Geometry check sheet. Reference: the model listing, model coordinates, mm. Face numbers are marked on the shaded views. A direction names the side the tool comes from. Round coordinates to 2 decimals unless told otherwise and drop trailing zeros. Write each loop counter-clockwise with the first axis right and the second up, starting at its lowest first coordinate (ties: lowest second). Pieces come first, ordered by that corner, then holes. Notation, with made-up numbers: (-28.5, -38.5) -> (15.5, -38.5) arc R14 cw to (15.5, -24.5) -> close; hole circle Ø7 at (28.25, -5). An arc over 180 degrees is marked (long way). Return JSON: item names as keys, results as strings. Group by question number.
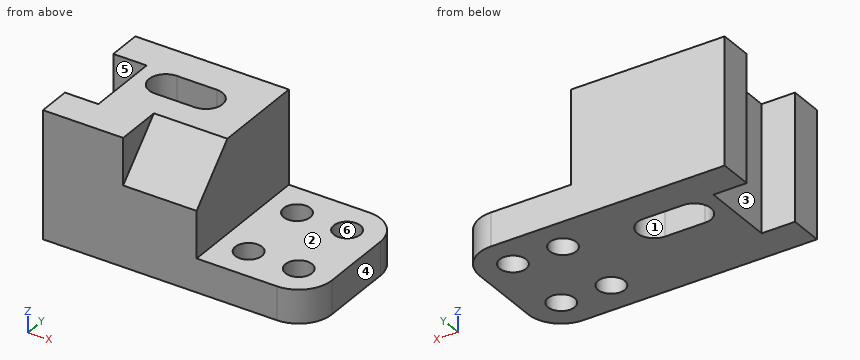
from build123d import *

# Parameters (mm, degrees)
SKETCH_W        = 80
SKETCH_H        = 42
PAD_DEPTH       = 38
SKETCH001_W     = 34
SKETCH001_H     = 42
POCKET_DEPTH    = 28
SKETCH002_W     = 10
SKETCH002_H     = 22
POCKET001_DEPTH = 38
SKETCH003_R     = 4
POCKET002_DEPTH = 38
POCKET003_DEPTH = 38
POCKET004_DEPTH = 22
FILLET_R        = 10
FILLET001_R     = 10


with BuildPart() as part:
    # Sketch → Pad (new body)
    with BuildSketch(Plane.XY):
        with Locations((40, 21)):
            Rectangle(SKETCH_W, SKETCH_H)
    extrude(amount=PAD_DEPTH)

    # Sketch001 (on Face6 of Pad) → Pocket (cut)
    with BuildSketch(Plane.XY.offset(38)):
        with Locations((63, 21)):
            Rectangle(SKETCH001_W, SKETCH001_H)
    extrude(amount=-POCKET_DEPTH, mode=Mode.SUBTRACT)

    # Sketch002 (on Face6 of Pocket) → Pocket001 (cut)
    with BuildSketch(Plane.XY.offset(38)):
        with Locations((5, 21)):
            Rectangle(SKETCH002_W, SKETCH002_H)
    extrude(amount=-POCKET001_DEPTH, mode=Mode.SUBTRACT)

    # Sketch003 (on Face6 of Pocket001) → Pocket002 (cut)
    with BuildSketch(Plane.XY.offset(38)):
        with Locations((55, 32)):
            Circle(SKETCH003_R)
        with Locations((70, 32)):
            Circle(SKETCH003_R)
        with Locations((55, 10)):
            Circle(SKETCH003_R)
        with Locations((70, 10)):
            Circle(SKETCH003_R)
    extrude(amount=-POCKET002_DEPTH, mode=Mode.SUBTRACT)

    # Sketch004 (on Face6 of Pocket002) → Pocket003 (cut)
    with BuildSketch(Plane.XY.offset(38)):
        with BuildLine():
            ThreePointArc((19, 32), (14, 27), (19, 22))
            Line((19, 22), (31, 22))
            ThreePointArc((31, 22), (35.99997, 27), (31, 32))
            Line((19, 32), (31, 32))
        make_face()
    extrude(amount=-POCKET003_DEPTH, mode=Mode.SUBTRACT)

    # Sketch005 (on Face5 of Pocket003) → Pocket004 (cut)
    with BuildSketch(Plane.YZ.offset(46)):
        Polygon((0, 24), (0, 38), (14, 38), align=None)
    extrude(amount=-POCKET004_DEPTH, mode=Mode.SUBTRACT)

    # Fillet
    fillet_edges = [part.edges().sort_by_distance(p)[0] for p in [
        (80, 0, 5),
    ]]
    fillet(fillet_edges, radius=FILLET_R)

    # Fillet001
    fillet001_edges = [part.edges().sort_by_distance(p)[0] for p in [
        (80, 42, 5),
    ]]
    fillet(fillet001_edges, radius=FILLET001_R)


solid = part.part
1) Sectioned sample at A-A on z = 11.5. Enter the section's corners in (x, y), and give its area (3 significant figures).
2) Sectioned sample at B-B on x = 55. Enter the section's corners in (y, z).
3) Sectioned sample at C-C on y = 27. Enter the section's corners in (x, z).
4) Sectioned sample at D-D on y = 20. Enter the section's corners in (x, z), and give its area (3 significant figures).
5) Tool access check on the marked faces 1, 2 and 3. Record the directions out of +Z, -Z, +X, -X, +Y, -Y that give a thin tool (end or side, any length) a straight path to the whole face; none if there is none.
6) Material ranges on probe 1 along Y at (x, z) = (70, 5); probe 2 along X at (y, z) = (11.5, 8.5); probe 3 along Z at (x, y) = (64.5, 3), recorded low to high. Write a range as [from, to].
7) Mould release check, pull along X, two halves, no side actions. Record for the marked faces 4, 5 and 6: +X half, -X half, draft (parallel to the pull), parting line (faces both ways), or undercut.
8) Go/stop test with flat-tipped pins: P1, Ø5, axis at y = 18.5, z = 20, coming from the -X side; P2, Ø12, axis at y = 21, z = 25.5, coming from the +X side; P3, Ø10.5, axis at x = 55, y = 10, coming from the +Z side. Record where each tip stops, or that it passes through.
Evaluation:
{
 "1": {"outline": "(0, 0) -> (46, 0) -> (46, 42) -> (0, 42) -> (0, 32) -> (10, 32) -> (10, 10) -> (0, 10) -> close; hole (19, 22) -> (31, 22) arc R5 ccw to (31, 32) -> (19, 32) arc R5 ccw to start", "area": "1,510 mm2"},
 "2": {"outline": "(0, 0) -> (6, 0) -> (6, 10) -> (0, 10) -> close; (14, 0) -> (28, 0) -> (28, 10) -> (14, 10) -> close; (36, 0) -> (42, 0) -> (42, 10) -> (36, 10) -> close"},
 "3": {"outline": "(10, 0) -> (14, 0) -> (14, 38) -> (10, 38) -> close; (36, 0) -> (80, 0) -> (80, 10) -> (46, 10) -> (46, 38) -> (36, 38) -> close"},
 "4": {"outline": "(10, 0) -> (80, 0) -> (80, 10) -> (46, 10) -> (46, 38) -> (10, 38) -> close", "area": "1,710 mm2"},
 "5": {"face 1": "+Z, -Z", "face 2": "+Z, +X, +Y, -Y", "face 3": "+Z, -Z, -X"},
 "6": {"probe 1": "y = [0, 6], [14, 28], [36, 42]", "probe 2": "x = [10, 51.29], [58.71, 66.29], [73.71, 80]", "probe 3": "z = [0, 10]"},
 "7": {"face 4": "+X half", "face 5": "draft", "face 6": "undercut"},
 "8": {"P1": "stops at x = 10", "P2": "stops at x = 46", "P3": "stops at z = 10"}
}
